from build123d import *

# Parameters (mm, degrees)
F0_W        = 45.72
F0_H        = 40.9903422
F1_DEPTH    = 5.08
F2_T1_DEPTH = 132.08
F4_DEPTH    = 25.4
F5_T1_DEPTH = 28.2903422
F5_T4_ANGLE = 112.9188061074
F5_T6_ANGLE = 112.9188061074


# Not quite as in the source:
# - a fillet or chamfer that OpenCascade refuses, or shapes differently, is made with other operations: its cross-section is extruded or revolved along the edge and cut away or added


with BuildPart() as f1:
    # F0 (on Top) → F1 (new body)
    with BuildSketch(Plane.XY):
        with Locations((22.86, 20.4951711)):
            Rectangle(F0_W, F0_H)
    extrude(amount=F1_DEPTH)

    # F2: fillet of radius 25.4 on 2 edges, made by hand

    # F2_s2 → F2_t1 (cut)
    with BuildSketch(Plane.XY.offset(-63.5)):
        with BuildLine():
            ThreePointArc((25.4, 40.9903422), (7.4394877579, 33.5508544421), (0, 15.5903422))
            Line((0, 15.5903422), (0, 40.9903422))
            Line((0, 40.9903422), (25.4, 40.9903422))
        make_face()
        with BuildLine():
            ThreePointArc((20.32, 40.9903422), (38.2805122421, 33.5508544421), (45.72, 15.5903422))
            Line((45.72, 15.5903422), (45.72, 40.9903422))
            Line((45.72, 40.9903422), (20.32, 40.9903422))
        make_face()
    extrude(amount=F2_T1_DEPTH, mode=Mode.SUBTRACT)

    # F3 (on face) → F4 (cut)
    with BuildSketch(Plane.XY.offset(5.08)):
        Polygon((5.343540106, 6.3080484979), (38.2127352059, 6.3080484979), (38.763590157, 21.9034794718), (37.315774709, 24.9750651419), (30.1536079496, 32.2724170983), (22.2911257297, 32.2724170983), (15.6609918922, 32.2724170983), (5.343540106, 20.2690735459), align=None)
    extrude(amount=-F4_DEPTH, mode=Mode.SUBTRACT)

    # F5: fillet of radius 5.08 on 4 edges, made by hand

    # F5_s2 → F5_t1 (cut)
    with BuildSketch(Plane.XZ.offset(-15.5903422)):
        with BuildLine():
            ThreePointArc((45.72, 0), (44.2321024484, 3.5921024484), (40.64, 5.08))
            Line((40.64, 5.08), (45.72, 5.08))
            Line((45.72, 5.08), (45.72, 0))
        make_face()
        with BuildLine():
            ThreePointArc((5.08, 5.08), (1.4878975516, 3.5921024484), (0, 0))
            Line((0, 0), (0, 5.08))
            Line((0, 5.08), (5.08, 5.08))
        make_face()
    extrude(amount=F5_T1_DEPTH, mode=Mode.SUBTRACT)

    # F5_s3 → F5_t4 (revolve, cut)
    with BuildSketch(Plane(origin=(22.8304215849, 9.6527795985, 0), x_dir=(0, 0, 1), z_dir=(-0.9210576344, -0.3894262885, 0))):
        with BuildLine():
            ThreePointArc((0, 31.8464615241), (3.5921024484, 30.3585639725), (5.08, 26.7664615241))
            Line((5.08, 26.7664615241), (5.08, 31.8464615241))
            Line((5.08, 31.8464615241), (0, 31.8464615241))
        make_face()
    revolve(axis=Axis((20.3199999999, 15.5903421999, 5.08), (0, 0, -1)), revolution_arc=F5_T4_ANGLE, mode=Mode.SUBTRACT)

    # F5_s5 → F5_t6 (revolve, cut)
    with BuildSketch(Plane.XZ.offset(-15.5903421999)):
        with BuildLine():
            ThreePointArc((5.08, 5.08), (1.4878975516, 3.5921024484), (0, 0))
            Line((0, 0), (0, 5.08))
            Line((0, 5.08), (5.08, 5.08))
        make_face()
    revolve(axis=Axis((25.4000000001, 15.5903421999, 5.08), (0, 0, -1)), revolution_arc=F5_T6_ANGLE, mode=Mode.SUBTRACT)


solid = f1.part
Here's how the part is built. I have some questions about the finished solid (model axes, mm). A direction names the side the tool comes from. Round coordinates to 2 decimals unless told otherwise and drop trailing zeros. Write each loop counter-clockwise with the first axis right and the second up, starting at its lowest first coordinate (ties: lowest second). Pieces come first, ordered by that corner, then holes.
1. For faces 4 (the flat face through (38.05, 23.42, 2.58)), 5 (the cylindrical face through (44.271, 7.904, 3.552)), which set-ups out of +Z, -Z, +X, -X, +Y, -Y let a thin tool reach every point of the face, with its end or its side?
2. Suppose I cut it at C-C (z = 1.8). List the corners of the cut face in (x, y) for me.
3. Will these pins go through, and if not, where does the flat tip stop? pin 1 Ø2 at (x, y) = (31, 37) entering from +Z; pin 2 Ø1.5 at (x, z) = (16, 1.5) entering from +Y; pin 3 Ø1.5 at (y, z) = (16.5, 3) entering from +X.
4. Suppose I cut it at A-A (z = 4.5). List the corners of the cut face in (x, y) for me.
5. Suppose I cut it at B-B (y = 15). List the corners of the cut face in (x, z) for me, and give its area (3 significant figures).
6. I need wall thicknesses on L1, parallel to Y at x = 12.5, z = 3.5; L2, parallel to X at y = 25, z = 0.9; L3, parallel to X at y = 28, z = 0.55. Which ranges of each line are inside material? Lowest first, please.
7. If we mould it in two halves opening along Y, with no side actions, what happens to faces 1 (the flat face through (23, 6, 5.08)), 2 (the flat face through (23, 32.272, 3)), 3 (the flat face through (23, 0, 3))? For each: released by +Y, released by -Y, zero draft, split by the parting line, or undercut.
Answer sheet:
1. face 4: +Z, -Z
1. face 5: +Z, +X, +Y, -Y
2. outline: (0.33, 0) - (45.39, 0) - (45.39, 15.59) arc R25.07 ccw to (22.86, 40.53) arc R25.07 ccw to (0.33, 15.59) - close; hole (5.34, 6.31) - (38.21, 6.31) - (38.76, 21.9) - (37.32, 24.98) - (30.15, 32.27) - (15.66, 32.27) - (5.34, 20.27) - close
3. pin 1: stops at z = 4.36
3. pin 2: stops at y = 39.3
3. pin 3: stops at x = 45.18
4. outline: (2.72, 0) - (43, 0) - (43, 15.59) arc R22.68 ccw to (22.86, 38.12) arc R22.68 ccw to (2.72, 15.59) - close; hole (5.34, 6.31) - (38.21, 6.31) - (38.76, 21.9) - (37.32, 24.98) - (30.15, 32.27) - (15.66, 32.27) - (5.34, 20.27) - close
5. outline: (0, 0) - (5.34, 0) - (5.34, 5.08) - (5.08, 5.08) arc R5.08 ccw to start; (38.52, 0) - (45.72, 0) arc R5.08 ccw to (40.64, 5.08) - (38.52, 5.08) - close
5. area: 52.6 mm2
6. L1: y = 0 to 6.31, 28.59 to 35.83
6. L2: x = 1.89 to 9.41, 37.29 to 43.83
6. L3: x = 3.27 to 11.99, 34.35 to 42.45
7. face 1: zero draft
7. face 2: undercut
7. face 3: released by -Y
